Input: part model. Units: mm. Frame: model coordinates. Face numbers are marked on the shaded views. A direction names the side the tool comes from. Round coordinates to 2 decimals unless told otherwise and drop trailing zeros. Write each loop counter-clockwise with the first axis right and the second up, starting at its lowest first coordinate (ties: lowest second). Pieces come first, ordered by that corner, then holes. Notation, with made-up numbers: (46.25, 17) -> (98.25, 17) arc R25 ccw to (98.25, 54) -> close; hole circle Ø10 at (40, -8.5). An arc over 180 degrees is marked (long way). Write item = value, one per line. Start each with the question number.
```python
from build123d import *

# Parameters (mm, degrees)
BOSS_EXTRUDE1_DEPTH = 5
CHAMFER1_SIZE       = 5
CUT_EXTRUDE1_DEPTH  = 3.5
SKETCH3_R           = 5
CUT_EXTRUDE2_DEPTH  = 0.75
CHAMFER2_SIZE       = 0.75
SKETCH4_R           = 1.875
SKETCH4_R_2         = 3.75
CUT_EXTRUDE3_DEPTH  = 48.326657393
SKETCH5_W           = 44
SKETCH5_H           = 3
BOSS_EXTRUDE2_DEPTH = 1.5
CHAMFER3_SIZE       = 1.5


with BuildPart() as part:
    # Sketch1 → Boss-Extrude1 (new body)
    with BuildSketch(Plane.XY):
        Polygon((37.25, 15), (44.75, 7.5), (44.75, -7.5), (37.25, -15), (-37.25, -15), (-37.25, 15), align=None)
    extrude(amount=BOSS_EXTRUDE1_DEPTH)

    # Chamfer1
    chamfer1_edges = [part.edges().sort_by_distance(p)[0] for p in [
        (-37.25, 0, 5),
    ]]
    chamfer(chamfer1_edges, length=CHAMFER1_SIZE - 0.0001)  # a hair under: the kernel refuses the full size

    # Sketch2 → Cut-Extrude1 (cut)
    with BuildSketch(Plane(origin=(0, 0, 0), x_dir=(-1, 0, 0), z_dir=(0, 0, -1))):
        with BuildLine():
            Line((-29.75, -11), (6.75, -11))
            ThreePointArc((6.75, -11), (17.75, 0), (6.75, 11))
            Line((6.75, 11), (-29.75, 11))
            ThreePointArc((-29.75, 11), (-40.75, 0), (-29.75, -11))
        make_face()
    extrude(amount=-CUT_EXTRUDE1_DEPTH, mode=Mode.SUBTRACT)

    # Sketch3 → Cut-Extrude2 (cut)
    with BuildSketch(Plane(origin=(0, 0, 3.5), x_dir=(-1, 0, 0), z_dir=(0, 0, -1))):
        with Locations((6.5, 0)):
            Circle(SKETCH3_R)
    extrude(amount=-CUT_EXTRUDE2_DEPTH, mode=Mode.SUBTRACT)

    # Chamfer2
    chamfer2_edges = [part.edges().sort_by_distance(p)[0] for p in [
        (-1.5, 0, 3.5),
    ]]
    chamfer(chamfer2_edges, length=CHAMFER2_SIZE - 0.0001)  # a hair under: the kernel refuses the full size

    # Sketch4 → Cut-Extrude3 (cut, through all)
    with BuildSketch(Plane(origin=(0, 0, 3.5), x_dir=(-1, 0, 0), z_dir=(0, 0, -1))):
        with Locations((-11.49, 0)):
            Circle(SKETCH4_R)
        with Locations((-29.75, 0)):
            Circle(SKETCH4_R_2)
    extrude(amount=-CUT_EXTRUDE3_DEPTH, mode=Mode.SUBTRACT)

    # Sketch5 → Boss-Extrude2 (add)
    with BuildSketch(Plane.XY.offset(5)):
        with Locations((-3, 9)):
            Rectangle(SKETCH5_W, SKETCH5_H)
        with BuildLine():
            Line((-25, 4.5), (19, 4.5))
            Line((19, 4.5), (19, 1.5))
            Line((19, 1.5), (14.088076211, 1.5))
            ThreePointArc((14.088076211, 1.5), (11.49, 3), (8.891923789, 1.5))
            Line((8.891923789, 1.5), (-25, 1.5))
            Line((-25, 1.5), (-25, 4.5))
        make_face()
        with Locations((-3, -9)):
            Rectangle(SKETCH5_W, SKETCH5_H)
        with BuildLine():
            Line((-25, -1.5), (8.891923789, -1.5))
            ThreePointArc((8.891923789, -1.5), (11.49, -3), (14.088076211, -1.5))
            Line((14.088076211, -1.5), (19, -1.5))
            Line((19, -1.5), (19, -4.5))
            Line((19, -4.5), (-25, -4.5))
            Line((-25, -4.5), (-25, -1.5))
        make_face()
    extrude(amount=BOSS_EXTRUDE2_DEPTH)

    # Chamfer3
    chamfer3_edges = [part.edges().sort_by_distance(p)[0] for p in [
        (-25, 9, 6.5),
        (-25, 3, 6.5),
        (-25, -3, 6.5),
        (-25, -9, 6.5),
        (19, -9, 6.5),
        (19, -3, 6.5),
        (19, 3, 6.5),
        (19, 9, 6.5),
    ]]
    chamfer(chamfer3_edges, length=CHAMFER3_SIZE - 0.0001)  # a hair under: the kernel refuses the full size


solid = part.part
```
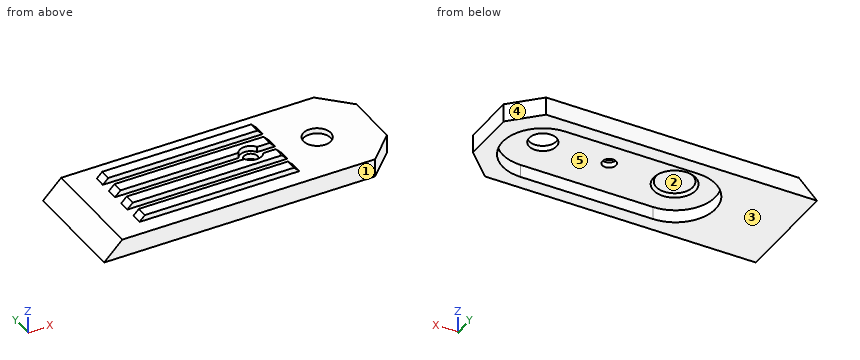
1. Mould query, pull axis X, two halves, no side actions, for the marked faces 3, 4 and 5. Classes: pulls with the +X half, pulls with the -X half, needs draft (parallel to the pull), parting line crosses it, or undercut.
2. Section C-C (z = 1.5). Output: boundary loops of the cut face in (x, y).
3. Section B-B (x = 11.49). Output: boundary loops of the cut face in (y, z) (3 decimals).
4. Pin query (flat end, axial travel): P1, Ø0.8, axis at x = -13, z = 5.5, coming from the +Y side; P2, Ø13, axis at x = -6.5, y = 0, coming from the -Z side; P3, Ø12, axis at x = 27, y = 7, coming from the +Z side. Return the tip coordinate at first contact, or that it passes through.
5. Section A-A (y = 0). State how many separate pieces and enclosed holes the cut face has, then the cut area to 3 significant figures.
6. Line query: line 1 along Y through (x, z) = (22, 2); line 2 along Y through (x, z) = (29.75, 4.45); line 3 along X through (y, z) = (2.5, 4). Output: solid intervals per line, ascending.
7. Section D-D (x = 38). Output: boundary loops of the cut face in (y, z), then the cut area to 3 significant figures.
8. Reachability of the marked faces 1 and 2 from +Z, -Z, +X, -X, +Y, -Y: full face, straight path, thin tool, end or side. Return the list, or none.
Check sheet entries:
q1.face_3 = needs draft
q1.face_4 = pulls with the +X half
q1.face_5 = undercut
q2.outline = (-35.75, -15) -> (37.25, -15) -> (44.75, -7.5) -> (44.75, 7.5) -> (37.25, 15) -> (-35.75, 15) -> close; hole (-6.75, -11) -> (29.75, -11) arc R11 ccw to (29.75, 11) -> (-6.75, 11) arc R11 ccw to start
q3.outline = (-15, 0) -> (-11, 0) -> (-11, 3.5) -> (-1.875, 3.5) -> (-1.875, 5) -> (-3, 5) -> (-3, 6.5) -> (-4.5, 6.5) -> (-4.5, 5) -> (-7.5, 5) -> (-7.5, 6.5) -> (-10.5, 6.5) -> (-10.5, 5) -> (-15, 5) -> close; (1.875, 3.5) -> (11, 3.5) -> (11, 0) -> (15, 0) -> (15, 5) -> (10.5, 5) -> (10.5, 6.5) -> (7.5, 6.5) -> (7.5, 5) -> (4.5, 5) -> (4.5, 6.5) -> (3, 6.5) -> (3, 5) -> (1.875, 5) -> close
q4.P1 = 10.5
q4.P2 = 3.5
q4.P3 = 5
q5.separate_pieces = 3
q5.enclosed_holes = 0
q5.area = 168 mm2
q6.line_1 = -15 to -11, 11 to 15
q6.line_2 = -15 to -3.75, 3.75 to 15
q6.line_3 = -33.25 to -11.12, -1.88 to 26.95, 32.55 to 44.75
q7.outline = (-14.25, 0) -> (-7.28, 0) -> (-7.28, 3.5) -> (7.28, 3.5) -> (7.28, 0) -> (14.25, 0) -> (14.25, 5) -> (-14.25, 5) -> close
q7.area = 91.6 mm2
q8.face_1 = +Z, -Z, +X, -X, -Y
q8.face_2 = -Z
